```python
from build123d import *

# Parameters (mm, degrees)
SKETCH2_W           = 54
SKETCH2_H           = 131
SKETCH2_W_2         = 32
SKETCH2_H_2         = 108
SKETCH12_W          = 54
SKETCH12_H          = 131
SKETCH12_W_2        = 32
SKETCH12_H_2        = 108
BOSS_EXTRUDE1_DEPTH = 1
SKETCH3_W           = 54
SKETCH3_H           = 135
SKETCH3_W_2         = 32
SKETCH3_H_2         = 108
EXTRUDE1_DEPTH      = 73
EXTRUDE2_REACH      = 763.64
SKETCH4_R           = 2.75
SKETCH4_W           = 108
SKETCH4_H           = 50
SKETCH7_W           = 54
SKETCH7_H           = 135
SKETCH7_W_2         = 32
SKETCH7_H_2         = 108
EXTRUDE5_DEPTH      = 73
EXTRUDE6_REACH      = 741.845
SKETCH8_R           = 2.75
SKETCH8_W           = 108
SKETCH8_H           = 50
SKETCH5_W           = 42
SKETCH5_H           = 36.5
EXTRUDE3_DEPTH      = 11.5
SKETCH6_W           = 42
SKETCH6_H           = 36.5
EXTRUDE4_DEPTH      = 11.5
SKETCH9_R           = 2.75
EXTRUDE7_DEPTH      = 7
SKETCH10_R          = 2.75
EXTRUDE8_DEPTH      = 7


with BuildPart() as part:
    # Sweep1: sweep along a path in Sketch1
    with BuildLine(Plane.XY) as sweep1_path:
        Line((-276, -375), (-276, -425))
        ThreePointArc((-276, -425), (-274.917785393, -441.412874927), (-271.689880586, -457.541553807))
        Line((-271.689880586, -457.541553807), (-245.689880586, -553.970166708))
        ThreePointArc((-245.689880586, -553.970166708), (-108.587125073, -645.346398294), (0, -521.428612901))
        Line((0, -521.428612901), (0, 0))
    # Sketch2 → Sweep1 (sweep)
    with BuildSketch(Plane(origin=(0, 0, 0), x_dir=(1, 0, 0), z_dir=(0, 1, 0))):
        with Locations((0, -65.5)):
            Rectangle(SKETCH2_W, SKETCH2_H)
        with Locations((0, -65.5)):
            Rectangle(SKETCH2_W_2, SKETCH2_H_2, mode=Mode.SUBTRACT)
    sweep(path=sweep1_path.line)

    # Sketch12 → Boss-Extrude1 (add)
    with BuildSketch(Plane(origin=(0, 0, 0), x_dir=(1, 0, 0), z_dir=(0, 1, 0))):
        with Locations((0, -65.5)):
            Rectangle(SKETCH12_W, SKETCH12_H)
        with Locations((0, -65.5)):
            Rectangle(SKETCH12_W_2, SKETCH12_H_2, mode=Mode.SUBTRACT)
    extrude(amount=BOSS_EXTRUDE1_DEPTH)

    # Sketch3 → Extrude1 (add)
    with BuildSketch(Plane(origin=(0, 1, 0), x_dir=(1, 0, 0), z_dir=(0, 1, 0))):
        with Locations((0, -65.5)):
            Rectangle(SKETCH3_W, SKETCH3_H)
        with Locations((0, -65.5)):
            Rectangle(SKETCH3_W_2, SKETCH3_H_2, mode=Mode.SUBTRACT)
    extrude(amount=EXTRUDE1_DEPTH)

    # Extrude2: up to this face of the body (flat: up to its plane)
    extrude2_end = Plane(part.part.faces().sort_by_distance((-27, -222.740088666, 65.5))[0])
    # Sketch4 → Extrude2 (cut, up to the picked face)
    with BuildSketch(Plane(origin=(27, 0, 0), x_dir=(0, 0, -1), z_dir=(1, 0, 0)), mode=Mode.PRIVATE) as extrude2_sk1:
        with Locations((-126.5, 61.5)):
            Circle(SKETCH4_R)
    extrude2_tool1 = split(extrude(extrude2_sk1.sketch, amount=-EXTRUDE2_REACH, mode=Mode.PRIVATE), bisect_by=extrude2_end, keep=Keep.BOTH, mode=Mode.PRIVATE)
    # Sketch4 → Extrude2 (cut, up to the picked face)
    with BuildSketch(Plane(origin=(27, 0, 0), x_dir=(0, 0, -1), z_dir=(1, 0, 0)), mode=Mode.PRIVATE) as extrude2_sk2:
        with Locations((-126.5, 39)):
            Circle(SKETCH4_R)
    extrude2_tool2 = split(extrude(extrude2_sk2.sketch, amount=-EXTRUDE2_REACH, mode=Mode.PRIVATE), bisect_by=extrude2_end, keep=Keep.BOTH, mode=Mode.PRIVATE)
    # Sketch4 → Extrude2 (cut, up to the picked face)
    with BuildSketch(Plane(origin=(27, 0, 0), x_dir=(0, 0, -1), z_dir=(1, 0, 0)), mode=Mode.PRIVATE) as extrude2_sk3:
        with Locations((-4.5, 39)):
            Circle(SKETCH4_R)
    extrude2_tool3 = split(extrude(extrude2_sk3.sketch, amount=-EXTRUDE2_REACH, mode=Mode.PRIVATE), bisect_by=extrude2_end, keep=Keep.BOTH, mode=Mode.PRIVATE)
    # Sketch4 → Extrude2 (cut, up to the picked face)
    with BuildSketch(Plane(origin=(27, 0, 0), x_dir=(0, 0, -1), z_dir=(1, 0, 0)), mode=Mode.PRIVATE) as extrude2_sk4:
        with Locations((-4.5, 61.5)):
            Circle(SKETCH4_R)
    extrude2_tool4 = split(extrude(extrude2_sk4.sketch, amount=-EXTRUDE2_REACH, mode=Mode.PRIVATE), bisect_by=extrude2_end, keep=Keep.BOTH, mode=Mode.PRIVATE)
    # Sketch4 → Extrude2 (cut, up to the picked face)
    with BuildSketch(Plane(origin=(27, 0, 0), x_dir=(0, 0, -1), z_dir=(1, 0, 0)), mode=Mode.PRIVATE) as extrude2_sk5:
        with Locations((-65.5, 49)):
            Rectangle(SKETCH4_W, SKETCH4_H)
    extrude2_tool5 = split(extrude(extrude2_sk5.sketch, amount=-EXTRUDE2_REACH, mode=Mode.PRIVATE), bisect_by=extrude2_end, keep=Keep.BOTH, mode=Mode.PRIVATE)
    add(extrude2_tool1.solids().sort_by(Axis((27, 61.5, 126.5), (-1, 0, 0)))[0], mode=Mode.SUBTRACT)
    add(extrude2_tool2.solids().sort_by(Axis((27, 39, 126.5), (-1, 0, 0)))[0], mode=Mode.SUBTRACT)
    add(extrude2_tool3.solids().sort_by(Axis((27, 39, 4.5), (-1, 0, 0)))[0], mode=Mode.SUBTRACT)
    add(extrude2_tool4.solids().sort_by(Axis((27, 61.5, 4.5), (-1, 0, 0)))[0], mode=Mode.SUBTRACT)
    add(extrude2_tool5.solids().sort_by(Axis((27, 49, 65.5), (-1, 0, 0)))[0], mode=Mode.SUBTRACT)

    # Sketch7 → Extrude5 (add)
    with BuildSketch(Plane(origin=(0, -375, 0), x_dir=(1, 0, 0), z_dir=(0, 1, 0))):
        with Locations((-276, -65.5)):
            Rectangle(SKETCH7_W, SKETCH7_H)
        with Locations((-276, -65.5)):
            Rectangle(SKETCH7_W_2, SKETCH7_H_2, mode=Mode.SUBTRACT)
    extrude(amount=EXTRUDE5_DEPTH)

    # Extrude6: up to this face of the body (flat: up to its plane)
    extrude6_end = Plane(part.part.faces().sort_by_distance((-303, -363.055013715, 65.5))[0])
    # Sketch8 → Extrude6 (cut, up to the picked face)
    with BuildSketch(Plane(origin=(-249, 0, 0), x_dir=(0, 0, -1), z_dir=(1, 0, 0)), mode=Mode.PRIVATE) as extrude6_sk1:
        with Locations((-4.5, -337)):
            Circle(SKETCH8_R)
    extrude6_tool1 = split(extrude(extrude6_sk1.sketch, amount=-EXTRUDE6_REACH, mode=Mode.PRIVATE), bisect_by=extrude6_end, keep=Keep.BOTH, mode=Mode.PRIVATE)
    # Sketch8 → Extrude6 (cut, up to the picked face)
    with BuildSketch(Plane(origin=(-249, 0, 0), x_dir=(0, 0, -1), z_dir=(1, 0, 0)), mode=Mode.PRIVATE) as extrude6_sk2:
        with Locations((-4.5, -314.5)):
            Circle(SKETCH8_R)
    extrude6_tool2 = split(extrude(extrude6_sk2.sketch, amount=-EXTRUDE6_REACH, mode=Mode.PRIVATE), bisect_by=extrude6_end, keep=Keep.BOTH, mode=Mode.PRIVATE)
    # Sketch8 → Extrude6 (cut, up to the picked face)
    with BuildSketch(Plane(origin=(-249, 0, 0), x_dir=(0, 0, -1), z_dir=(1, 0, 0)), mode=Mode.PRIVATE) as extrude6_sk3:
        with Locations((-126.5, -337)):
            Circle(SKETCH8_R)
    extrude6_tool3 = split(extrude(extrude6_sk3.sketch, amount=-EXTRUDE6_REACH, mode=Mode.PRIVATE), bisect_by=extrude6_end, keep=Keep.BOTH, mode=Mode.PRIVATE)
    # Sketch8 → Extrude6 (cut, up to the picked face)
    with BuildSketch(Plane(origin=(-249, 0, 0), x_dir=(0, 0, -1), z_dir=(1, 0, 0)), mode=Mode.PRIVATE) as extrude6_sk4:
        with Locations((-126.5, -314.5)):
            Circle(SKETCH8_R)
    extrude6_tool4 = split(extrude(extrude6_sk4.sketch, amount=-EXTRUDE6_REACH, mode=Mode.PRIVATE), bisect_by=extrude6_end, keep=Keep.BOTH, mode=Mode.PRIVATE)
    # Sketch8 → Extrude6 (cut, up to the picked face)
    with BuildSketch(Plane(origin=(-249, 0, 0), x_dir=(0, 0, -1), z_dir=(1, 0, 0)), mode=Mode.PRIVATE) as extrude6_sk5:
        with Locations((-65.5, -327)):
            Rectangle(SKETCH8_W, SKETCH8_H)
    extrude6_tool5 = split(extrude(extrude6_sk5.sketch, amount=-EXTRUDE6_REACH, mode=Mode.PRIVATE), bisect_by=extrude6_end, keep=Keep.BOTH, mode=Mode.PRIVATE)
    add(extrude6_tool1.solids().sort_by(Axis((-249, -337, 4.5), (-1, 0, 0)))[0], mode=Mode.SUBTRACT)
    add(extrude6_tool2.solids().sort_by(Axis((-249, -314.5, 4.5), (-1, 0, 0)))[0], mode=Mode.SUBTRACT)
    add(extrude6_tool3.solids().sort_by(Axis((-249, -337, 126.5), (-1, 0, 0)))[0], mode=Mode.SUBTRACT)
    add(extrude6_tool4.solids().sort_by(Axis((-249, -314.5, 126.5), (-1, 0, 0)))[0], mode=Mode.SUBTRACT)
    add(extrude6_tool5.solids().sort_by(Axis((-249, -327, 65.5), (-1, 0, 0)))[0], mode=Mode.SUBTRACT)

    # Sketch5 → Extrude3 (cut)
    with BuildSketch(Plane.XY.offset(133)):
        with Locations((0, 49.75)):
            Rectangle(SKETCH5_W, SKETCH5_H)
        with Locations((-276, -326.25)):
            Rectangle(SKETCH5_W, SKETCH5_H)
    extrude(amount=-EXTRUDE3_DEPTH, mode=Mode.SUBTRACT)

    # Sketch6 → Extrude4 (cut)
    with BuildSketch(Plane(origin=(0, 0, -2), x_dir=(-1, 0, 0), z_dir=(0, 0, -1))):
        with Locations((0, 49.75)):
            Rectangle(SKETCH6_W, SKETCH6_H)
        with Locations((276, -326.25)):
            Rectangle(SKETCH6_W, SKETCH6_H)
    extrude(amount=-EXTRUDE4_DEPTH, mode=Mode.SUBTRACT)

    # Sketch9 → Extrude7 (cut)
    with BuildSketch(Plane(origin=(0, 74, 0), x_dir=(1, 0, 0), z_dir=(0, 1, 0))):
        with Locations(Location((-11, -126.5, 0), (0, 0, 180))):
            Circle(SKETCH9_R)
        with Locations(Location((11, -126.5, 0), (0, 0, 180))):
            Circle(SKETCH9_R)
        with Locations(Location((11, -4.5, 0), (0, 0, 180))):
            Circle(SKETCH9_R)
        with Locations(Location((-11, -4.5, 0), (0, 0, 180))):
            Circle(SKETCH9_R)
    extrude(amount=-EXTRUDE7_DEPTH, mode=Mode.SUBTRACT)

    # Sketch10 → Extrude8 (cut)
    with BuildSketch(Plane(origin=(0, -302, 0), x_dir=(1, 0, 0), z_dir=(0, 1, 0))):
        with Locations(Location((-287, -126.5, 0), (0, 0, 270))):
            Circle(SKETCH10_R)
        with Locations(Location((-265, -126.5, 0), (0, 0, 270))):
            Circle(SKETCH10_R)
        with Locations(Location((-287, -4.5, 0), (0, 0, 270))):
            Circle(SKETCH10_R)
        with Locations(Location((-265, -4.5, 0), (0, 0, 270))):
            Circle(SKETCH10_R)
    extrude(amount=-EXTRUDE8_DEPTH, mode=Mode.SUBTRACT)


solid = part.part
```
Design review of the part built by this model. Coordinates are the model's own, in mm. A direction names the side the tool comes from. Give positions to 0.01 mm unless a question says otherwise; leave off trailing zeros. Write each loop counter-clockwise with the first axis right and the second up, starting at its lowest first coordinate (ties: lowest second). Pieces come first, ordered by that corner, then holes. Notation, with made-up numbers: (-5, 63.5) -> (24, 63.5) arc R14 ccw to (24, 68.5) -> close; hole circle Ø1 at (79, -23). An arc over 180 degrees is marked (long way). Answer in a Markdown table with one row per item.
(1) Clearance check with flat-ended pins moving along their axes: pin 1 (6 mm diameter, centred on x = -5, z = 127, fed in from -Y); pin 2 (3.5 mm diameter, centred on x = -287, z = 126.5, fed in from +Y); pin 3 (4 mm diameter, centred on x = -268, z = 114.5, fed in from -Y). State where each tip first meets the part, or that it passes through.
Results:
| item | result |
|---|---|
| pin 1 | y = -618.46 |
| pin 2 | y = -344.5 |
| pin 3 | y = -578.2 |
(2) Consider section B-B (z = 72). State the section outline as (x, y) points, then the cut area to 3 significant figures.
Results:
| item | result |
|---|---|
| outline | (-303, -425) arc R152 ccw to (-297.76, -464.57) -> (-271.76, -561) arc R152 ccw to (27, -521.43) -> (27, 24) -> (16, 24) -> (16, -521.43) arc R141 cw to (-261.14, -558.14) -> (-287.14, -461.71) arc R141 cw to (-292, -425) -> (-292, -352) -> (-303, -352) -> close; (-260, -425) arc R109 ccw to (-256.24, -453.38) -> (-230.24, -549.8) arc R109 ccw to (-16, -521.43) -> (-16, 24) -> (-27, 24) -> (-27, -521.43) arc R98 cw to (-219.62, -546.94) -> (-245.62, -450.51) arc R98 cw to (-249, -425) -> (-249, -352) -> (-260, -352) -> close |
| area | 24,400 mm2 |
(3) Consider section A-A (y = -398.5). State the section outline as (x, z) points.
Results:
| item | result |
|---|---|
| outline | (-303, 0) -> (-249, 0) -> (-249, 131) -> (-303, 131) -> close; (-27, 0) -> (27, 0) -> (27, 131) -> (-27, 131) -> close; hole (-292, 11.5) -> (-260, 11.5) -> (-260, 119.5) -> (-292, 119.5) -> close; hole (-16, 11.5) -> (16, 11.5) -> (16, 119.5) -> (-16, 119.5) -> close |
(4) Consider section C-C (y = -198). State the section outline as (x, z) points.
Results:
| item | result |
|---|---|
| outline | (-27, 0) -> (27, 0) -> (27, 131) -> (-27, 131) -> close; hole (-16, 11.5) -> (16, 11.5) -> (16, 119.5) -> (-16, 119.5) -> close |
(5) Mouldability with a two-part tool opening along X and no side actions: class faces 1 (the flat face through (0, 29, -2)), 2 (the cylindrical face through (-108.082, -672.484, 64.583)), 3 (the flat face through (-249, -378, 66)) as +X half, -X half, draft (parallel to the pull), parting line (faces both ways), or undercut.
Results:
| item | result |
|---|---|
| face 1 | draft |
| face 2 | parting line |
| face 3 | undercut |
(6) Consider section D-D (x = -237). State the section outline as (y, z) points, then the cut area to 3 significant figures.
Results:
| item | result |
|---|---|
| outline | (-624.19, 0) -> (-482.49, 0) -> (-482.49, 131) -> (-624.19, 131) -> close; hole (-607.08, 11.5) -> (-524.74, 11.5) -> (-524.74, 119.5) -> (-607.08, 119.5) -> close |
| area | 9,670 mm2 |
(7) For faces 4 (the flat face through (-276, -302, 5)), 5 (the flat face through (-15, -350, 119.5)), 6 (the flat face through (-27, -228, 66)), 7 (the cylindrical face through (-290.813, -443.256, 66.256)), list the 3-axis set-ups (+Z, -Z, +X, -X, +Y, -Y) from which the entire face can be reached by the end or side of a thin tool; tool diameter is ignored.
Results:
| item | result |
|---|---|
| face 4 | +Z, -Z, -X, +Y |
| face 5 | none |
| face 6 | +Z, -Z, +Y |
| face 7 | +Y |
(8) To check wall thickness, follow probe 1 along X at (y, z) = (-386, 115); probe 2 along Z at (x, y) = (-252.6, -337); probe 3 along X at (y, z) = (-306.3, 4.5). State the ranges of each line that lie inside material, in increasing order.
Results:
| item | result |
|---|---|
| probe 1 | -303 to -292, -260 to -249, -27 to -16, 16 to 27 |
| probe 2 | -2 to 1.75, 7.25 to 11.5, 119.5 to 123.75, 129.25 to 133 |
| probe 3 | -303 to -289.75, -284.25 to -267.75, -262.25 to -249, -27 to 27 |
